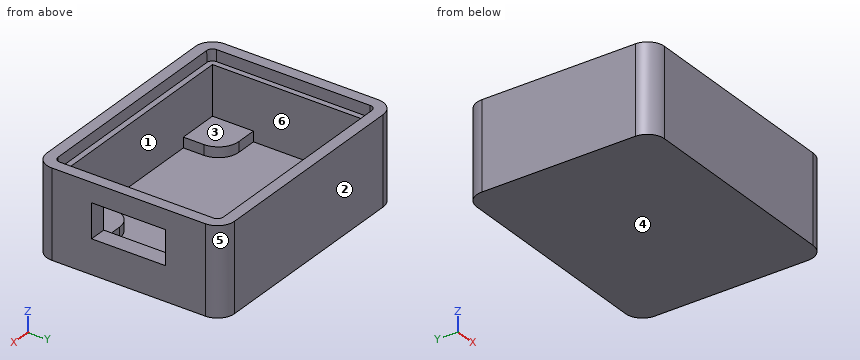
from build123d import *

# Parameters (mm, degrees)
SKETCH1_W           = 27
SKETCH1_H           = 36.7
BOSS_EXTRUDE1_DEPTH = 10.4
SHELL1_T            = 3
BOSS_EXTRUDE2_DEPTH = 1.8
CUT_EXTRUDE1_REACH  = 48.944
SKETCH3_W           = 13
SKETCH3_H           = 6
FILLET1_R           = 3
LIP2_START          = 10.4
LIP2_DEPTH          = 2


with BuildPart() as part:
    # Sketch1 → Boss-Extrude1 (new body)
    with BuildSketch(Plane(origin=(0, 0, 0), x_dir=(0, 1, 0), z_dir=(0, 0, 1))):
        Rectangle(SKETCH1_W, SKETCH1_H)
    extrude(amount=BOSS_EXTRUDE1_DEPTH)

    # Shell1
    shell1_openings = [part.faces().sort_by_distance(p)[0] for p in [
        (0, 0, 10.4),
    ]]
    offset(amount=SHELL1_T, openings=shell1_openings, kind=Kind.INTERSECTION)

    # Sketch2 → Boss-Extrude2 (add)
    with BuildSketch(Plane.XY):
        with BuildLine():
            Line((-11.15, 9.9), (-11.15, 13.5))
            Line((-11.15, 13.5), (-18.35, 13.5))
            Line((-18.35, 13.5), (-18.35, 6.3))
            Line((-18.35, 6.3), (-14.75, 6.3))
            ThreePointArc((-14.75, 6.3), (-12.204415588, 7.354415588), (-11.15, 9.9))
        make_face()
        with BuildLine():
            Line((18.35, 13.5), (11.15, 13.5))
            Line((11.15, 13.5), (11.15, 9.9))
            ThreePointArc((11.15, 9.9), (12.204415588, 7.354415588), (14.75, 6.3))
            Line((14.75, 6.3), (18.35, 6.3))
            Line((18.35, 6.3), (18.35, 13.5))
        make_face()
        with BuildLine():
            Line((18.35, -13.5), (18.35, -6.3))
            Line((18.35, -6.3), (14.75, -6.3))
            ThreePointArc((14.75, -6.3), (12.204415588, -7.354415588), (11.15, -9.9))
            Line((11.15, -9.9), (11.15, -13.5))
            Line((11.15, -13.5), (18.35, -13.5))
        make_face()
        with BuildLine():
            Line((-14.75, -6.3), (-18.35, -6.3))
            Line((-18.35, -6.3), (-18.35, -13.5))
            Line((-18.35, -13.5), (-11.15, -13.5))
            Line((-11.15, -13.5), (-11.15, -9.9))
            ThreePointArc((-11.15, -9.9), (-12.204415588, -7.354415588), (-14.75, -6.3))
        make_face()
    extrude(amount=BOSS_EXTRUDE2_DEPTH)

    # Sketch3 → Cut-Extrude1 (cut, up to next)
    with BuildSketch(Plane.YZ.offset(21.35), mode=Mode.PRIVATE) as cut_extrude1_sk1:
        with Locations((0, 6)):
            Rectangle(SKETCH3_W, SKETCH3_H)
    cut_extrude1_tool1 = extrude(cut_extrude1_sk1.sketch, amount=-CUT_EXTRUDE1_REACH, mode=Mode.PRIVATE) & part.part
    add(cut_extrude1_tool1.solids().sort_by_distance((21.35, 0, 6))[0], mode=Mode.SUBTRACT)

    # Fillet1
    fillet1_edges = [part.edges().sort_by_distance(p)[0] for p in [
        (21.35, 16.5, 3.7),
        (21.35, -16.5, 3.7),
        (-21.35, -16.5, 3.7),
        (-21.35, 16.5, 3.7),
    ]]
    fillet(fillet1_edges, radius=FILLET1_R)

    # Lip2: read off the stored shape, not the designer's step
    # Lip2 outline → Lip2 (add)
    with BuildSketch(Plane.XY.offset(LIP2_START)):
        with BuildLine():
            Line((18.35, 16.5), (-18.35, 16.5))
            ThreePointArc((-18.35, 16.5), (-20.471320344, 15.621320344), (-21.35, 13.5))
            Line((-21.35, 13.5), (-21.35, -13.5))
            ThreePointArc((-21.35, -13.5), (-20.471320344, -15.621320344), (-18.35, -16.5))
            Line((-18.35, -16.5), (18.35, -16.5))
            ThreePointArc((18.35, -16.5), (20.471320344, -15.621320344), (21.35, -13.5))
            Line((21.35, -13.5), (21.35, 13.5))
            ThreePointArc((21.35, 13.5), (20.471320344, 15.621320344), (18.35, 16.5))
        make_face()
    extrude(amount=LIP2_DEPTH)

    # Lip2 2: loft between two sections, ruled curve by curve
    lip2_2_from = [
        Edge.make_three_point_arc((18.35, -14.5, 10.4), (19.057106781, -14.207106781, 10.4), (19.35, -13.5, 10.4)),
        Edge.make_three_point_arc((-19.35, -13.5, 10.4), (-19.057106781, -14.207106781, 10.4), (-18.35, -14.5, 10.4)),
        Edge.make_three_point_arc((-18.35, 14.5, 10.4), (-19.057106781, 14.207106781, 10.4), (-19.35, 13.5, 10.4)),
        Edge.make_three_point_arc((19.35, 13.5, 10.4), (19.057106781, 14.207106781, 10.4), (18.35, 14.5, 10.4)),
        Edge.make_line((19.35, -13.5, 10.4), (19.35, 13.5, 10.4)),
        Edge.make_line((-18.35, -14.5, 10.4), (18.35, -14.5, 10.4)),
        Edge.make_line((-19.35, 13.5, 10.4), (-19.35, -13.5, 10.4)),
        Edge.make_line((18.35, 14.5, 10.4), (-18.35, 14.5, 10.4)),
    ]
    lip2_2_to = [
        Edge.make_three_point_arc((18.35, -14.517453736, 12.4), (19.069448436, -14.219448436, 12.4), (19.367453736, -13.5, 12.4)),
        Edge.make_three_point_arc((-19.367453736, -13.5, 12.4), (-19.069448436, -14.219448436, 12.4), (-18.35, -14.517453736, 12.4)),
        Edge.make_three_point_arc((-18.35, 14.517453736, 12.4), (-19.069448436, 14.219448436, 12.4), (-19.367453736, 13.5, 12.4)),
        Edge.make_three_point_arc((19.367453736, 13.5, 12.4), (19.069448436, 14.219448436, 12.4), (18.35, 14.517453736, 12.4)),
        Edge.make_line((19.367453736, -13.5, 12.4), (19.367453736, 13.5, 12.4)),
        Edge.make_line((-18.35, -14.517453736, 12.4), (18.35, -14.517453736, 12.4)),
        Edge.make_line((-19.367453736, 13.5, 12.4), (-19.367453736, -13.5, 12.4)),
        Edge.make_line((18.35, 14.517453736, 12.4), (-18.35, 14.517453736, 12.4)),
    ]
    lip2_2 = Solid(Shell([*[Face.make_surface_from_curves(lip2_2_from[k], lip2_2_to[k]) for k in range(8)], Face(Wire(lip2_2_from)), Face(Wire(lip2_2_to))]))
    add(lip2_2, mode=Mode.SUBTRACT)


solid = part.part
The model under review builds one solid part; all positions refer to its coordinate system, in mm. Face numbers are marked on the shaded views. A direction names the side the tool comes from. Give positions to 0.01 mm unless a question says otherwise; leave off trailing zeros. Write each loop counter-clockwise with the first axis right and the second up, starting at its lowest first coordinate (ties: lowest second). Pieces come first, ordered by that corner, then holes.
1. Add section B-B, the plane z = 5. Write out the cut boundary in (x, y), plus the area to 3 significant figures.
2. Wall thickness on L1, parallel to X at y = 7, z = 3.5; L2, parallel to Y at x = -16.5, z = 6.75; L3, parallel to Y at x = -7.5, z = 11: over which ranges is each line inside the solid? List them lowest first.
3. Add section A-A, the plane z = 9.75. Write out the cut boundary in (x, y), plus the area to 3 significant figures.
4. Tool access review of the marked faces 1 and 2: name each direction out of +Z, -Z, +X, -X, +Y, -Y from which nothing blocks a thin tool from reaching the whole face with its end or side.
5. For P1, Ø3.5, axis at x = -13.5, y = 11, coming from the +Z side; P2, Ø0.9, axis at x = 20, z = 7, coming from the -Y side, all flat-tipped, find the tip position at first contact; note any pin that passes through.
6. Draft analysis for pull direction X (two halves, no side actions). For the marked faces 3, 4, 5 and 6, state which applies: +X half, -X half, draft (parallel to the pull), parting line (faces both ways), or undercut.
Worked answers:
1. outline: (-21.35, -13.5) arc R3 ccw to (-18.35, -16.5) - (18.35, -16.5) arc R3 ccw to (21.35, -13.5) - (21.35, -6.5) - (18.35, -6.5) - (18.35, -13.5) - (-18.35, -13.5) - (-18.35, 13.5) - (18.35, 13.5) - (18.35, 6.5) - (21.35, 6.5) - (21.35, 13.5) arc R3 ccw to (18.35, 16.5) - (-18.35, 16.5) arc R3 ccw to (-21.35, 13.5) - close
1. area: 371 mm2
2. L1: x = -21.35 to -18.35, 18.35 to 21.35
2. L2: y = -16.5 to -13.5, 13.5 to 16.5
2. L3: y = -16.5 to -14.51, 14.51 to 16.5
3. outline: (-21.35, -13.5) arc R3 ccw to (-18.35, -16.5) - (18.35, -16.5) arc R3 ccw to (21.35, -13.5) - (21.35, 13.5) arc R3 ccw to (18.35, 16.5) - (-18.35, 16.5) arc R3 ccw to (-21.35, 13.5) - close; hole (-18.35, -13.5) - (18.35, -13.5) - (18.35, 13.5) - (-18.35, 13.5) - close
3. area: 410 mm2
4. face 1: +Z
4. face 2: +Z, -Z, +X, -X, +Y
5. P1: stops at z = 1.8
5. P2: stops at y = -16.25
6. face 3: undercut
6. face 4: draft
6. face 5: +X half
6. face 6: undercut
